Study the drawing (mm; zero at the part's minimum x, y, z) and answer. Give positions to 0.01 mm unless a question says otherwise; leave off trailing zeros. Write each loop counter-clockwise with the first axis right and the second up, starting at its lowest first coordinate (ties: lowest second). Pieces come first, ordered by that corner, then holes. Notation, with made-up numbers: (75.5, 81.25) - (93.5, 81.25) arc R31 cw to (93.5, 114.25) - close; hole circle Ø2 at (-28.5, 22.25). An arc over 180 degrees is marked (long way). Return JSON: item names as keys, results as strings.
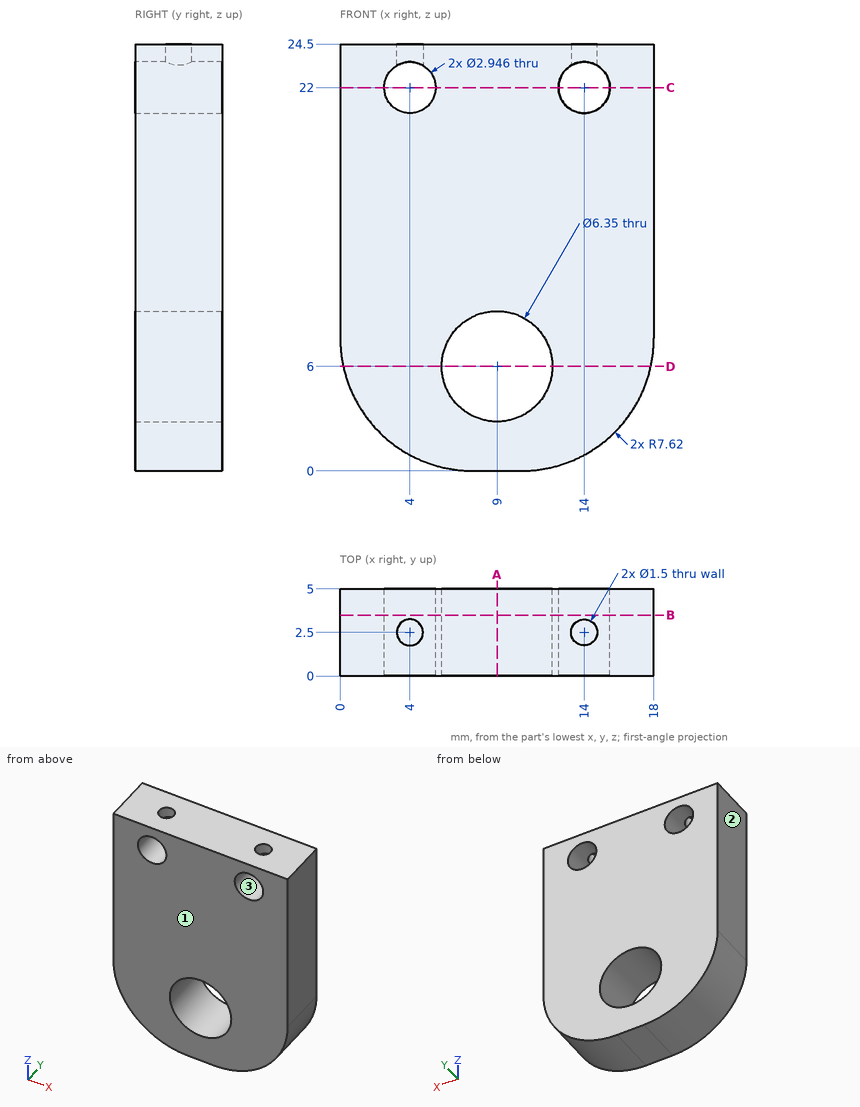
Item 1: A cutting plane is placed at C-C on z = 22. Determine the outline of the cut face in (x, y).
Answer below:
{"outline": "(0, 0) - (2.53, 0) - (2.53, 5) - (0, 5) - close; (5.47, 0) - (12.53, 0) - (12.53, 5) - (5.47, 5) - close; (15.47, 0) - (18, 0) - (18, 5) - (15.47, 5) - close"}
Item 2: A cutting plane is placed at B-B on y = 3.5. Give the number of separate pieces and of enclosed holes in the cut face, then the cut area to 3 significant figures.
Answer below:
{"separate pieces": "1", "enclosed holes": "3", "area": "371 mm²"}
Item 3: Flat-ended cylindrical pins translate along their axes: P1, Ø1.8, axis at x = 4, z = 22, coming from the -Y side; P2, Ø1.2, axis at x = 14, y = 2.5, coming from the -Z side. Find the tip coordinate at first contact, or state that the pin passes through.
Answer below:
{"P1": "passes through", "P2": "stops at z = 0.62"}
Item 4: A cutting plane is placed at A-A on x = 9. Determine the outline of the cut face in (y, z) (1 decimal).
Answer below:
{"outline": "(0, 0) - (5, 0) - (5, 2.8) - (0, 2.8) - close; (0, 9.2) - (5, 9.2) - (5, 24.5) - (0, 24.5) - close"}
Item 5: Consider L1, parallel to X at y = 1.3, z = 22; L2, parallel to Y at x = 4, z = 24; L3, parallel to Z at x = 10.5, y = 0.65. Determine where each line is inside the solid, lowest interval first.
Answer below:
{"L1": "x = 0 to 2.53, 5.47 to 12.53, 15.47 to 18", "L2": "y = 0 to 1.75, 3.25 to 5", "L3": "z = 0 to 3.2, 8.8 to 24.5"}
Item 6: The mould has two halves that part along X. Classify the marked faces 1, 2 and 3: +X half, -X half, draft (parallel to the pull), parting line (faces both ways), or undercut.
Answer below:
{"face 1": "draft", "face 2": "-X half", "face 3": "undercut"}
Item 7: A cutting plane is placed at D-D on z = 6. Determine the outline of the cut face in (x, y) (1 decimal), then the cut area to 3 significant figures.
Answer below:
{"outline": "(0.2, 0) - (5.8, 0) - (5.8, 5) - (0.2, 5) - close; (12.2, 0) - (17.8, 0) - (17.8, 5) - (12.2, 5) - close", "area": "56.5 mm²"}
